from build123d import *

# Parameters (mm, degrees)
F0_W     = 50.8
F0_H     = 76.2
F1_DEPTH = 12.7
F2_W     = 50.8
F2_H     = 12.7
F3_DEPTH = 25.4
F4_W     = 12.7
F4_H     = 12.7
F5_DEPTH = 12.7
F6_R     = 12.7
F7_DEPTH = 12.701


with BuildPart() as f1:
    # F0 (on Top) → F1 (new body)
    with BuildSketch(Plane.XY):
        Rectangle(F0_W, F0_H)
    extrude(amount=F1_DEPTH)

    # F2 (on face) → F3 (join)
    with BuildSketch(Plane.XY.offset(12.7)):
        with Locations((0, 31.75)):
            Rectangle(F2_W, F2_H)
    extrude(amount=F3_DEPTH)

    # F4 (on face) → F5 (cut)
    with BuildSketch(Plane.XY.offset(38.1)):
        with Locations((-19.05, 31.75)):
            Rectangle(F4_W, F4_H)
    extrude(amount=-F5_DEPTH, mode=Mode.SUBTRACT)

    # F6 (on face) → F7 (cut, through all)
    with BuildSketch(Plane.XY.offset(12.7)):
        with Locations((0, -12.7)):
            Circle(F6_R)
        with BuildLine():
            ThreePointArc((-2.54e-08, -38.1), (-17.9605122511, -30.6605122332), (-25.4, -12.7))
            Line((-25.4, -12.7), (-25.4, -38.1))
            Line((-25.4, -38.1), (-2.54e-08, -38.1))
        make_face()
        with BuildLine():
            ThreePointArc((25.4, -12.7), (17.9605122332, -30.6605122511), (-2.54e-08, -38.1))
            Line((-2.54e-08, -38.1), (25.4, -38.1))
            Line((25.4, -38.1), (25.4, -12.7))
        make_face()
    extrude(amount=-F7_DEPTH, mode=Mode.SUBTRACT)


solid = f1.part
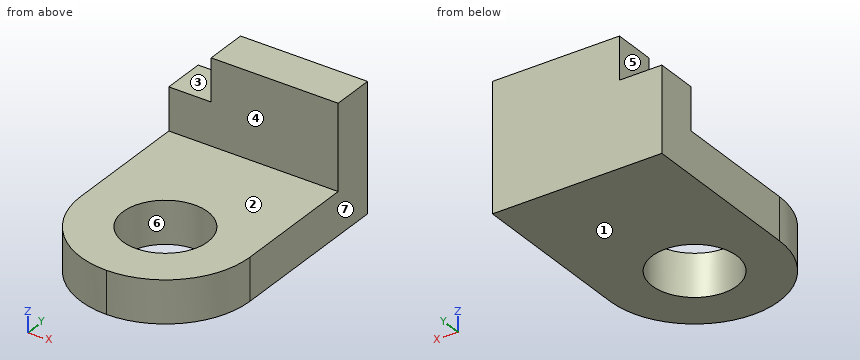
Here's how the part is built. I have some questions about the finished solid (model axes, mm). Face numbers are marked on the shaded views. A direction names the side the tool comes from. Round coordinates to 2 decimals unless told otherwise and drop trailing zeros. Loops run counter-clockwise (first coordinate to the right, second up) from the corner with the lowest first, then second, coordinate; pieces in that order, holes last. Notation, with made-up numbers: (-33, 55) - (-9, 55) arc R10 ccw to (-9, 61) - close; hole circle Ø8 at (-25.5, 10). An arc over 180 degrees is marked (long way). One line per question, with ' | ' between items. Start each with the question number.
Q1. Please list where these lines run through material, in increasing order: line 1 (Y direction, x = 0, z = 4.75); line 2 (Z direction, x = -18, y = 25.5); line 3 (Y direction, x = 21, z = 34). Write a range as [from, to].
Q2. We'd pull the mould along X, two halves only. Please class the marked faces 4, 5, 6 and 7: +X half, -X half, draft (parallel to the pull), parting line (faces both ways), or undercut.
Q3. I want a section at D-D (y = 28). Write out the boundary of the cut face in (x, z), then the cut area to 3 significant figures.
Q4. For the marked faces 1, 2 and 3, which set-ups out of +Z, -Z, +X, -X, +Y, -Y let a thin tool reach every point of the face, with its end or its side?
Q5. Will these pins go through, and if not, where does the flat tip stop? pin 1 (20.5 mm diameter, centred on x = -12, z = 24.5, fed in from -Y); pin 2 (20.5 mm diameter, centred on x = 0, y = -12.7, fed in from +Z); pin 3 (8 mm diameter, centred on x = -5, z = 15.5, fed in from -Y); pin 4 (14 mm diameter, centred on y = 34, z = 34.5, fed in from -X).
Q6. I want a section at B-B (x = -7). Write out the boundary of the cut face in (y, z).
Q7. I want a section at A-A (y = -19). Write out the boundary of the cut face in (x, z), then the cut area to 3 significant figures.
Q8. I want a section at C-C (z = 11.5). Write out the boundary of the cut face in (x, y), then the cut area to 3 significant figures.
Response values:
1) line 1: y = [-38.1, -25.4], [0, 38.1] | line 2: z = [0, 25.4] | line 3: y = [25.4, 38.1]
2) face 4: draft | face 5: -X half | face 6: undercut | face 7: +X half
3) outline: (-25.4, 0) - (25.4, 0) - (25.4, 38.1) - (-12.7, 38.1) - (-12.7, 25.4) - (-25.4, 25.4) - close | area: 1,770 mm²
4) face 1: -Z, +X, -X, +Y, -Y | face 2: +Z, +X, -X, -Y | face 3: +Z, -X, +Y, -Y
5) pin 1: stops at y = 25.4 | pin 2: passes through | pin 3: stops at y = -38.01 | pin 4: stops at x = -12.7
6) outline: (-37.12, 0) - (-23.3, 0) - (-23.3, 12.7) - (-37.12, 12.7) - close; (-2.1, 0) - (38.1, 0) - (38.1, 38.1) - (25.4, 38.1) - (25.4, 12.7) - (-2.1, 12.7) - close
7) outline: (-24.61, 0) - (-11.03, 0) - (-11.03, 12.7) - (-24.61, 12.7) - close; (11.03, 0) - (24.61, 0) - (24.61, 12.7) - (11.03, 12.7) - close | area: 345 mm²
8) outline: (-25.4, -12.7) arc R25.4 ccw to (25.4, -12.7) - (25.4, 38.1) - (-25.4, 38.1) - close; hole circle Ø25.4 at (0, -12.7) | area: 3,090 mm²
